Read the model definition and answer for the solid it produces. Units are mm, in the model's axes. A direction names the side the tool comes from. Coordinates: 2 decimals unless noted, no trailing zeros. Write each loop counter-clockwise with the first axis right and the second up, starting at its lowest first coordinate (ties: lowest second). Pieces come first, ordered by that corner, then holes. Notation, with made-up numbers: (-6.5, 14.5) -> (4.5, 14.5) arc R17 cw to (4.5, 31.5) -> close; hole circle Ø11 at (-34.5, -34). An arc over 180 degrees is marked (long way). Answer in a Markdown table with one row per item. Add a question column.
Item 1: Given pin 1 Ø6.5 at (x, z) = (-211.201, -80.01) entering from -Y; pin 2 Ø10.5 at (x, z) = (-26, 46.5) entering from +Y, each flat-ended and moving along its own axis, determine where each tip first touches the part or whether it passes through.
Item 2: Section B-B on z = -127 is taken. Write down the section's boundary in (x, y), then the cut area to 3 significant figures.
Item 3: Straight lines are drawn through the part: line 1 (Z direction, x = 27.85, y = 21.5); line 2 (X direction, y = 7, z = -80.01); line 3 (Z direction, x = -27.85, y = 9.5). For each, find the intervals that lie inside material, in ascending order. Write a range as from..to.
Item 4: Section A-A on x = -27.85 is taken. Write down the section's boundary in (y, z).
Item 5: Which of the six approach directions +Z, -Z, +X, -X, +Y, -Y give full straight-line access (tool end or side, diameter ignored) to faces 1 (the face through (205.955, 13.023, 125.348)), 2 (the face through (53, 19.566, -5))?
Item 6: For a pull along X with two mould halves and no side action, classify faces 3 (the face through (-3, 26.416, -3)), 4 (the face through (-241.3, 13, 3)), 5 (the face through (-45.779, 23.039, 4.113)) as +X half, -X half, draft (parallel to the pull), parting line (faces both ways), or undercut.
Item 7: Section C-C on x = 55.7 is taken. Write down the section's boundary in (y, z).
```python
from build123d import *

# Parameters (mm, degrees)
SKETCH1_W                                = 482.6
SKETCH1_H                                = 406.4
BOSS_EXTRUDE1_DEPTH                      = 26.416
SKETCH3_R                                = 1.27
SKETCH3_R_2                              = 5.25
CUT_EXTRUDE2_DEPTH                       = 27.416
CBORE_FOR_M10_HEX_HEAD_BOLT1_D           = 11
CBORE_FOR_M10_HEX_HEAD_BOLT1_CBORE_D     = 21.48
CBORE_FOR_M10_HEX_HEAD_BOLT1_CBORE_DEPTH = 6.85
M10_CLEARANCE_HOLE1_D                    = 11


with BuildPart() as part:
    # Sketch1 → Boss-Extrude1 (new body)
    with BuildSketch(Plane(origin=(0, 0, 0), x_dir=(1, 0, 0), z_dir=(0, 1, 0))):
        Rectangle(SKETCH1_W, SKETCH1_H)
    extrude(amount=BOSS_EXTRUDE1_DEPTH)

    # Sketch3 → Cut-Extrude2 (cut, through all)
    with BuildSketch(Plane(origin=(0, 26.416, 0), x_dir=(1, 0, 0), z_dir=(0, 1, 0))):
        with Locations((-211.201, -80.01)):
            Circle(SKETCH3_R)
        with Locations((-211.201, 80.01)):
            Circle(SKETCH3_R)
        with Locations((211.201, -80.01)):
            Circle(SKETCH3_R)
        with Locations((211.201, 80.01)):
            Circle(SKETCH3_R)
        with Locations((55.7, 0)):
            Circle(SKETCH3_R_2)
        with Locations((27.85, -48.237614991)):
            Circle(SKETCH3_R_2)
        with Locations((-27.85, -48.237614991)):
            Circle(SKETCH3_R_2)
        with Locations((-55.7, 0)):
            Circle(SKETCH3_R_2)
        with Locations((-27.85, 48.237614991)):
            Circle(SKETCH3_R_2)
        with Locations((27.85, 48.237614991)):
            Circle(SKETCH3_R_2)
        with Locations((-211.201, -127)):
            Circle(SKETCH3_R)
        with Locations((211.201, -127)):
            Circle(SKETCH3_R)
        with Locations((211.201, 127)):
            Circle(SKETCH3_R)
        with Locations((-211.201, 127)):
            Circle(SKETCH3_R)
    extrude(amount=-CUT_EXTRUDE2_DEPTH, mode=Mode.SUBTRACT)

    # CBORE for M10 Hex Head Bolt1 (through all)
    with Locations(Plane(origin=(0, 26.416, 0), x_dir=(1, 0, 0), z_dir=(0, 1, 0))):
        with Locations((27.85, 48.237614991), (55.7, 0), (27.85, -48.237614991), (-27.85, -48.237614991), (-55.7, 0), (-27.85, 48.237614991)):
            CounterBoreHole(CBORE_FOR_M10_HEX_HEAD_BOLT1_D / 2, CBORE_FOR_M10_HEX_HEAD_BOLT1_CBORE_D / 2, CBORE_FOR_M10_HEX_HEAD_BOLT1_CBORE_DEPTH)

    # M10 Clearance Hole1 (through all)
    with Locations(Plane(origin=(0, 26.416, 0), x_dir=(1, 0, 0), z_dir=(0, 1, 0))):
        with Locations((-211.201, 127), (-211.201, 80.01), (-211.201, -80.01), (-211.201, -127), (211.201, -127), (211.201, -80.01), (211.201, 80.01), (211.201, 127)):
            Hole(M10_CLEARANCE_HOLE1_D / 2)


solid = part.part
```
Results below:
| question | item | result |
|---|---|---|
| 1 | pin 1 | passes through |
| 1 | pin 2 | stops at y = 19.57 |
| 2 | outline | (-241.3, 0) -> (-216.7, 0) -> (-216.7, 26.42) -> (-241.3, 26.42) -> close; (-205.7, 0) -> (205.7, 0) -> (205.7, 26.42) -> (-205.7, 26.42) -> close; (216.7, 0) -> (241.3, 0) -> (241.3, 26.42) -> (216.7, 26.42) -> close |
| 2 | area | 12,200 mm2 |
| 3 | line 1 | z = -203.2..-58.98, -37.5..37.5, 58.98..203.2 |
| 3 | line 2 | x = -241.3..-216.7, -205.7..205.7, 216.7..241.3 |
| 3 | line 3 | z = -203.2..-53.74, -42.74..42.74, 53.74..203.2 |
| 4 | outline | (0, -203.2) -> (26.42, -203.2) -> (26.42, -58.98) -> (19.57, -58.98) -> (19.57, -53.74) -> (0, -53.74) -> close; (0, -42.74) -> (19.57, -42.74) -> (19.57, -37.5) -> (26.42, -37.5) -> (26.42, 37.5) -> (19.57, 37.5) -> (19.57, 42.74) -> (0, 42.74) -> close; (0, 53.74) -> (19.57, 53.74) -> (19.57, 58.98) -> (26.42, 58.98) -> (26.42, 203.2) -> (0, 203.2) -> close |
| 5 | face 1 | +Y, -Y |
| 5 | face 2 | +Y |
| 6 | face 3 | draft |
| 6 | face 4 | -X half |
| 6 | face 5 | undercut |
| 7 | outline | (0, -203.2) -> (26.42, -203.2) -> (26.42, -10.74) -> (19.57, -10.74) -> (19.57, -5.5) -> (0, -5.5) -> close; (0, 5.5) -> (19.57, 5.5) -> (19.57, 10.74) -> (26.42, 10.74) -> (26.42, 203.2) -> (0, 203.2) -> close |
